from build123d import *

# Parameters (mm, degrees)
F0_R     = 4
F1_DEPTH = 1
F2_R     = 3
F3_DEPTH = 6
F6_W     = 2
F6_H     = 12.68074
F6_W_2   = 1.971088
F6_H_2   = 12.97379
F6_W_3   = 1.876695
F6_H_3   = 11.885081
F7_DEPTH = 12.5
F8_R     = 1
F9_DEPTH = 6.001


with BuildPart() as f1:
    # F0 (on Top) → F1 (new body)
    with BuildSketch(Plane.XY):
        Circle(F0_R)
    extrude(amount=F1_DEPTH)

    # F2 (on face) → F3 (join)
    with BuildSketch(Plane.XY.offset(1)):
        Circle(F2_R)
    extrude(amount=F3_DEPTH)

    # F4 (on Front) → F5 (revolve)
    with BuildSketch(Plane.XZ):
        with BuildLine():
            Line((0, 7), (3, 7))
            ThreePointArc((3, 7), (2.12132, 9.12132), (0, 10))
            Line((0, 10), (0, 7))
        make_face()
    revolve(axis=Axis((0, 0, 8.5), (0, 0, -1)))

    # F6 (on Front) → F7 (cut, symmetric)
    with BuildSketch(Plane.XZ):
        with Locations((0, 9.34037)):
            Rectangle(F6_W, F6_H)
        with Locations((2.985544, 9.486895)):
            Rectangle(F6_W_2, F6_H_2)
        with Locations((-2.938347, 8.94254)):
            Rectangle(F6_W_3, F6_H_3)
    extrude(amount=F7_DEPTH, both=True, mode=Mode.SUBTRACT)

    # F8 (on face) → F9 (cut, through all)
    with BuildSketch(Plane(origin=(-2, 0, 0), x_dir=(0, -1, 0), z_dir=(-1, 0, 0))):
        with Locations((0, 7)):
            Circle(F8_R)
    extrude(amount=-F9_DEPTH, mode=Mode.SUBTRACT)


solid = f1.part
Geometry: final body of the model. Coordinates: model frame, mm. A direction names the side the tool comes from. Give positions to 0.01 mm unless a question says otherwise; leave off trailing zeros. Loops run counter-clockwise (first coordinate to the right, second up) from the corner with the lowest first, then second, coordinate; pieces in that order, holes last. Notation, with made-up numbers: (46, -38) - (75, -38) arc R5 cw to (75, -32) - close; hole circle Ø6 at (87.5, 24.25). An arc over 180 degrees is marked (long way). Answer as CSV lines item,"result". Start each with the question number.
1. Section B-B, the plane x = 0. Return loops of the section in (y, z), plus the area to 3 significant figures.
2. Reachability of faces 5 (the face through (1, 0, 5.6)), 6 (the face through (1, 3, 1)), 7 (the face through (2.4, 0, 3)) from +Z, -Z, +X, -X, +Y, -Y: full face, straight path, thin tool, end or side. Return the list, or none.
3. Section C-C, the plane y = 0. Give the number of separate pieces and of enclosed holes in the cut face, plus the area to 3 significant figures.
4. Draft query along Y for faces 1 (the face through (-1.51, 0.13, 7.99)), 2 (the face through (0, 0, 3)), 3 (the face through (-0.867, -3.905, 0.493)), 4 (the face through (1.49, 0.13, 7.99)). Return one class per face: released by +Y, released by -Y, zero draft, split by the parting line, or undercut.
5. Ray query, L1, parallel to X at y = 1.25, z = 7.5; L2, parallel to Z at x = -2.5, y = 2.25; L3, parallel to Z at x = -1.8, y = 0. Return the intervals inside material, ascending.
6. Pin query (flat end, axial travel): P1, Ø1.3, axis at y = 0, z = 6, coming from the +X side; P2, Ø4, axis at y = -1.5, z = 2.5, coming from the +X side; P3, Ø2, axis at x = -0.5, z = 2.5, coming from the -Y side. Return the tip coordinate at first contact, or that it passes through.
7. Section A-A, the plane z = 4. Return loops of the section in (x, y), plus the area to 3 significant figures.
Answers:
1,outline,"(-4, 0) - (4, 0) - (4, 1) - (3, 1) - (3, 3) - (-3, 3) - (-3, 1) - (-4, 1) - close"
1,area,"20.0 mm2"
2,face 5,"+Z, +Y, -Y"
2,face 6,"+Z"
2,face 7,"+Z, +X, +Y, -Y"
3,separate pieces,"3"
3,enclosed holes,"0"
3,area,"29.2 mm2"
4,face 1,"undercut"
4,face 2,"zero draft"
4,face 3,"split by the parting line"
4,face 4,"undercut"
5,L1,"x = -2 to -1, 1 to 2"
5,L2,"z = 0 to 1"
5,L3,"z = 0 to 6, 8 to 9.4"
6,P1,"stops at x = 2"
6,P2,"stops at x = 4"
6,P3,"stops at y = -3"
7,outline,"(-2, -2.24) arc R3 ccw to (-1, -2.83) - (-1, 2.83) arc R3 ccw to (-2, 2.24) - close; (1, -2.83) arc R3 ccw to (2, -2.24) - (2, 2.24) arc R3 ccw to (1, 2.83) - close"
7,area,"10.3 mm2"
